For this review, take the finished solid that the model builds, in its own axes (mm). Face numbers are marked on the shaded views. A direction names the side the tool comes from. Round coordinates to 2 decimals unless told otherwise and drop trailing zeros. Write each loop counter-clockwise with the first axis right and the second up, starting at its lowest first coordinate (ties: lowest second). Pieces come first, ordered by that corner, then holes. Notation, with made-up numbers: (-23.75, 81) -> (35.25, 81) arc R34 ccw to (35.25, 118) -> close; hole circle Ø4 at (52, 66). An arc over 180 degrees is marked (long way). Write item = value, one per line. Start each with the question number.
```python
from build123d import *

# Parameters (mm, degrees)
F1_DEPTH = 25
F0_W     = 21
F0_H     = 46
F2_DEPTH = 2
F3_W     = 8
F3_H     = 50
F4_DEPTH = 20
F5_W     = 5.5
F5_H     = 11
F6_DEPTH = 15
F7_W     = 6
F7_H     = 11
F8_DEPTH = 44.5
F9_SIZE  = 1.99999


# Not quite as in the source:
# - a fillet or chamfer is up to 0.001 mm smaller than in the source, because OpenCascade refuses the exact size


with BuildPart() as f1:
    # F0 (on Top) → F1 (new body)
    with BuildSketch(Plane.XY):
        Polygon((0, 25), (0, 23), (0, -23), (0, -25), (8, -25), (8, 25), align=None)
        Polygon((-21, 23), (0, 23), (0, 25), (-23, 25), (-23, -25), (0, -25), (0, -23), (-21, -23), align=None)
    extrude(amount=F1_DEPTH)

    # F0 (on Top) → F2 (join)
    with BuildSketch(Plane.XY):
        Polygon((0, 25), (0, 23), (0, -23), (0, -25), (8, -25), (8, 25), align=None)
        with Locations((-10.5, 0)):
            Rectangle(F0_W, F0_H)
        Polygon((-21, 23), (0, 23), (0, 25), (-23, 25), (-23, -25), (0, -25), (0, -23), (-21, -23), align=None)
    extrude(amount=F2_DEPTH)

    # F3 (on face) → F4 (join)
    with BuildSketch(Plane.XY.offset(25)):
        with Locations((4, 0)):
            Rectangle(F3_W, F3_H)
    extrude(amount=F4_DEPTH)

    # F5 (on face) → F6 (join)
    with BuildSketch(Plane.YZ.offset(8)):
        with Locations((-22.25, 39.5)):
            Rectangle(F5_W, F5_H)
    extrude(amount=F6_DEPTH)

    # F7 (on face) → F8 (join, through all)
    with BuildSketch(Plane(origin=(0, -19.5, 0), x_dir=(-1, 0, 0), z_dir=(0, 1, 0))):
        with Locations((-20, 39.5)):
            Rectangle(F7_W, F7_H)
    extrude(amount=F8_DEPTH)

    # F9 (size 2 in the source; OpenCascade refuses exactly that, so slightly less here)
    f9_edges = [f1.edges().sort_by_distance(p)[0] for p in [
        (-10.5, 23, 25),
        (-21, 0, 25),
        (-10.5, -23, 25),
        (0, 0, 45),
    ]]
    chamfer(f9_edges, length=F9_SIZE)


solid = f1.part
```
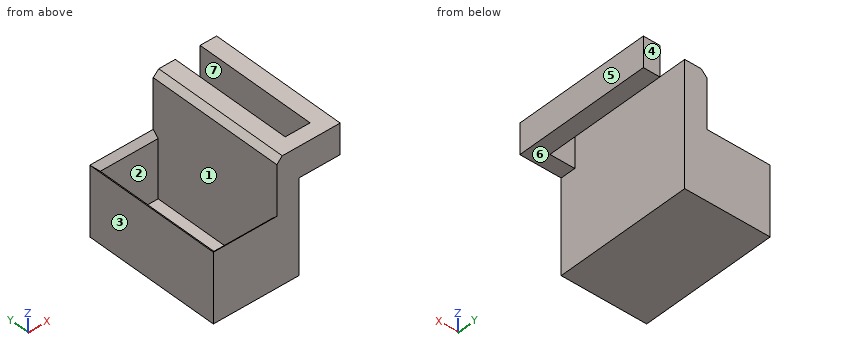
1. Machinability: for the marked faces 5, 6 and 7, which of the approach directions +Z, -Z, +X, -X, +Y, -Y give a long, thin tool a straight path to every point of the face, cutting with its end or side? Answer none if there is none.
2. Consider section B-B, the plane z = 39.5. Give the boundary of the cut face in (x, y).
3. Consider section D-D, the plane z = 3. Give the boundary of the cut face in (x, y), then the cut area to 3 significant figures.
4. Clearance check with flat-ended pins moving along their axes: pin 1 Ø10.5 at (y, z) = (-7, 14.5) entering from +X; pin 2 Ø4.5 at (x, z) = (10.5, 42) entering from +Y; pin 3 Ø12 at (x, y) = (-6.5, 3) entering from +Z. State where each tip first meets the part, or that it passes through.
5. Draft analysis for pull direction X (two halves, no side actions). For the marked faces 1, 2, 3 and 4, state which applies: +X half, -X half, draft (parallel to the pull), parting line (faces both ways), or undercut.
6. Wall thickness on L1, parallel to X at y = -18.5, z = 18; L2, parallel to Y at x = -12, z = 19.5; L3, parallel to X at y = 19, z = 42.5: over which ranges is each line inside the solid? List them lowest first. Write a range as from..to.
Outcome:
q1.face_5 = +Z, -Z, +X, +Y, -Y
q1.face_6 = -Z, +X, +Y, -Y
q1.face_7 = +Z, -Z, +Y
q2.outline = (0, -25) -> (23, -25) -> (23, 25) -> (17, 25) -> (17, -19.5) -> (8, -19.5) -> (8, 25) -> (0, 25) -> close
q3.outline = (-23, -25) -> (8, -25) -> (8, 25) -> (-23, 25) -> close; hole (-21, -23) -> (0, -23) -> (0, 23) -> (-21, 23) -> close
q3.area = 584 mm2
q4.pin_1 = 8
q4.pin_2 = -19.5
q4.pin_3 = 2
q5.face_1 = undercut
q5.face_2 = undercut
q5.face_3 = -X half
q5.face_4 = draft
q6.L1 = -23..-21, 0..8
q6.L2 = -25..-23, 23..25
q6.L3 = 0..8, 17..23
